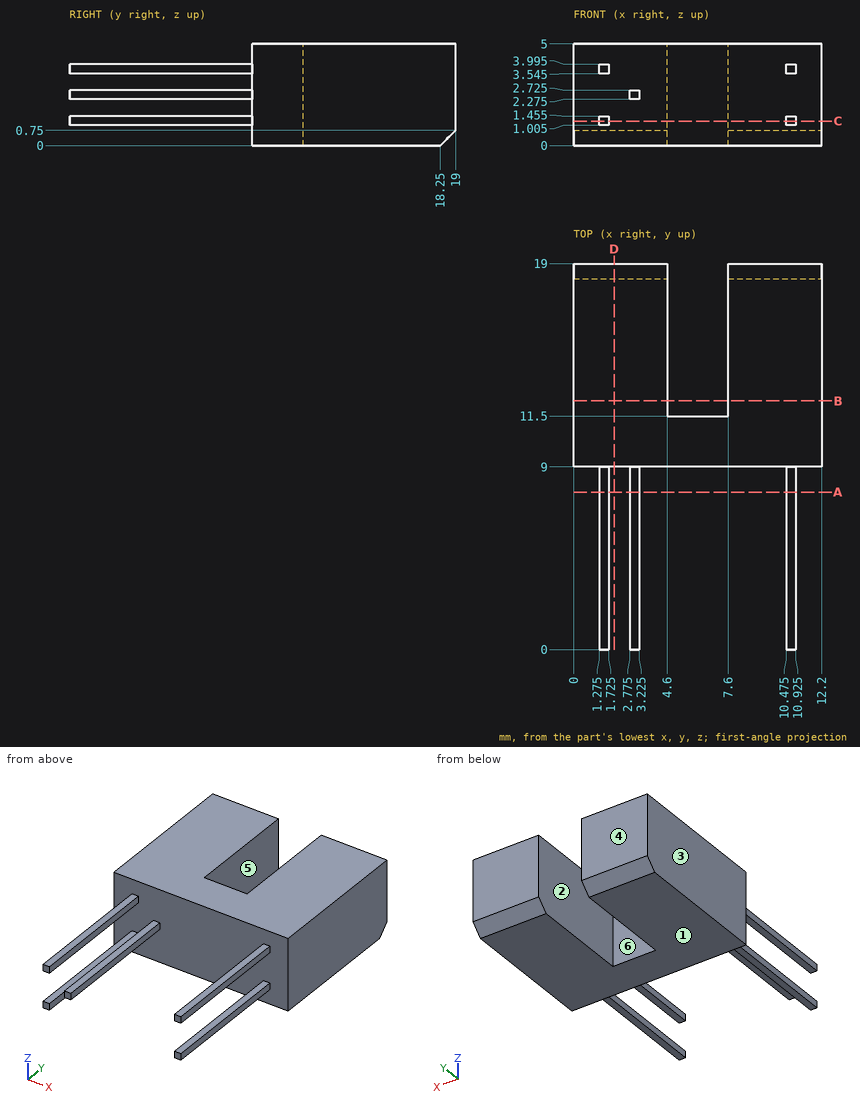
Source: three-view drawing plus pictorial views. Frame: mm from the lowest corner of the part. A direction names the side the tool comes from. Give positions to 0.01 mm unless a question says otherwise; leave off trailing zeros. Loops run counter-clockwise (first coordinate to the right, second up) from the corner with the lowest first, then second, coordinate; pieces in that order, holes last. Notation, with made-up numbers: M -9.75,29.25 L 7.25,29.25 A25 ccw 7.25,46.25 Z; hole C 6.5,78.5 d4. An arc over 180 degrees is marked long. Put each result on its own line as item: value.
Q1. Mould query, pull axis X, two halves, no side actions, for the marked faces 3, 4, 5 and 6. Classes: released by +X, released by -X, zero draft, split by the parting line, or undercut.
Response values:
face 3: released by -X
face 4: zero draft
face 5: undercut
face 6: undercut
Q2. Line query: probe 1 along X at (y, z) = (18.25, 3.65); probe 2 along X at (y, z) = (6.25, 3.8) (3 decimals); probe 3 along Y at (x, z) = (6.25, 2.05). Output: solid intervals per line, ascending. Write a range as [from, to].
Response values:
probe 1: x = [0, 4.6], [7.6, 12.2]
probe 2: x = [1.275, 1.725], [10.475, 10.925]
probe 3: y = [9, 11.5]
Q3. Section B-B (y = 12.25). Return the cut outline in (x, z).
Response values:
outline: M 0,0 L 4.6,0 L 4.6,5 L 0,5 Z; M 7.6,0 L 12.2,0 L 12.2,5 L 7.6,5 Z
Q4. Section A-A (y = 7.75). Return the cut outline in (x, z) (3 decimals), and give its area (3 significant figures).
Response values:
outline: M 1.275,1.005 L 1.725,1.005 L 1.725,1.455 L 1.275,1.455 Z; M 1.275,3.545 L 1.725,3.545 L 1.725,3.995 L 1.275,3.995 Z; M 2.775,2.275 L 3.225,2.275 L 3.225,2.725 L 2.775,2.725 Z; M 10.475,1.005 L 10.925,1.005 L 10.925,1.455 L 10.475,1.455 Z; M 10.475,3.545 L 10.925,3.545 L 10.925,3.995 L 10.475,3.995 Z
area: 1.01 mm²
Q5. Reachability of the marked faces 1 and 2 from +Z, -Z, +X, -X, +Y, -Y: full face, straight path, thin tool, end or side. Return the list, or none.
Response values:
face 1: -Z, +X, -X, +Y, -Y
face 2: +Z, -Z, +Y
Q6. Section D-D (x = 2). Return the cut outline in (y, z), and give its area (3 significant figures).
Response values:
outline: M 9,0 L 18.25,0 L 19,0.75 L 19,5 L 9,5 Z
area: 49.7 mm²
Q7. Pin query (flat end, axial travel): P1, Ø0.5, axis at x = 10.5, y = 5, coming from the +Z side (3 decimals); P2, Ø1, axis at x = 2, z = 4.5, coming from the -Y side; P3, Ø0.5, axis at y = 3, z = 4, coming from the -X side (3 decimals). Return the tip coordinate at first contact, or that it passes through.
Response values:
P1: stops at z = 3.995
P2: stops at y = 9
P3: stops at x = 1.275
Q8. Section C-C (z = 1.2). Return the cut outline in (x, y) (3 decimals), and give its area (3 significant figures).
Response values:
outline: M 0,9 L 1.275,9 L 1.275,0 L 1.725,0 L 1.725,9 L 10.475,9 L 10.475,0 L 10.925,0 L 10.925,9 L 12.2,9 L 12.2,19 L 7.6,19 L 7.6,11.5 L 4.6,11.5 L 4.6,19 L 0,19 Z
area: 108 mm²
